Geometry: final body of the model. Coordinates: model frame, mm. Face numbers are marked on the shaded views. A direction names the side the tool comes from. Give positions to 0.01 mm unless a question says otherwise; leave off trailing zeros. Loops run counter-clockwise (first coordinate to the right, second up) from the corner with the lowest first, then second, coordinate; pieces in that order, holes last. Notation, with made-up numbers: (8.5, 41) - (53.5, 41) arc R11 cw to (53.5, 61) - close; hole circle Ø6 at (32, 41.5). An arc over 180 degrees is marked (long way). Use one line per item in the form item = value.
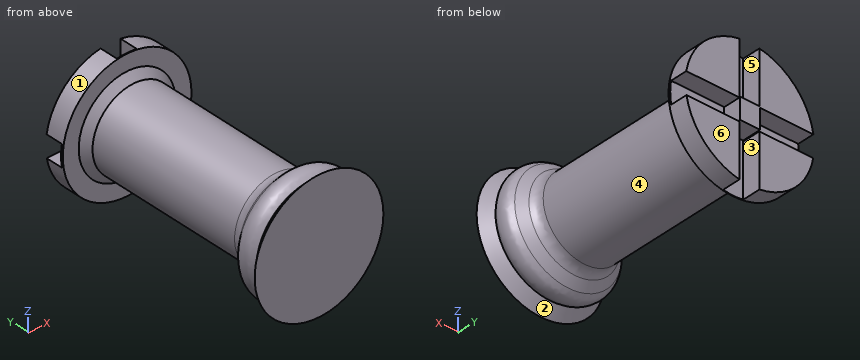
```python
from build123d import *

# Parameters (mm, degrees)
F2_R     = 5.08
F3_SIZE  = 2.54
F4_W     = 6.907339
F4_H     = 51.517231
F5_DEPTH = 6.35
F6_W     = 52.092841
F6_H     = 7.48295
F7_DEPTH = 5.9436
F8_W     = 6.907339
F8_H     = 7.284426
F9_DEPTH = 6.604


with BuildPart() as f1:
    # F0 (on Top) → F1 (revolve)
    with BuildSketch(Plane.XY):
        Polygon((22.304947, 47.919661), (0, 47.919661), (0, -33.52937), (22.304947, -33.52937), (18.717232, -30.197919), (22.304947, -26.334228), (14.246386, -18.851276), (14.246386, 41.300129), (22.304947, 41.300129), align=None)
    revolve(axis=Axis((0, 7.195146, 0), (0, -1, 0)))

    # F2
    f2_edges = [f1.edges().sort_by_distance(p)[0] for p in [
        (-22.304947, -26.334228, 0),
        (-14.246386, -18.851276, 0),
    ]]
    fillet(f2_edges, radius=F2_R)

    # F3
    f3_edges = [f1.edges().sort_by_distance(p)[0] for p in [
        (14.246386, 12.332043, 0),
        (-14.246383, -16.636044, 0),
        (-14.246386, 41.300129, 0),
    ]]
    chamfer(f3_edges, length=F3_SIZE)

    # F4 (on face) → F5 (cut)
    with BuildSketch(Plane(origin=(0, 47.919661, 0), x_dir=(-1, 0, 0), z_dir=(0, 1, 0))):
        with Locations((-0.143903, 0.575613)):
            Rectangle(F4_W, F4_H)
    extrude(amount=-F5_DEPTH, mode=Mode.SUBTRACT)

    # F6 (on face) → F7 (cut)
    with BuildSketch(Plane(origin=(0, 47.919661, 0), x_dir=(-1, 0, 0), z_dir=(0, 1, 0))):
        with Locations((0.287805, -0.143903)):
            Rectangle(F6_W, F6_H)
    extrude(amount=-F7_DEPTH, mode=Mode.SUBTRACT)

    # F8 (on face) → F9 (join)
    with BuildSketch(Plane(origin=(0, 41.569661, 0), x_dir=(-1, 0, 0), z_dir=(0, 1, 0))):
        with Locations((-0.143903, 0.12047)):
            Rectangle(F8_W, F8_H)
    extrude(amount=F9_DEPTH)


solid = f1.part
```
(1) Material intervals for L1, parallel to Y at x = -1, z = 6.5; L2, parallel to Y at x = -19, z = 2.5; L3, parallel to Y at x = -11.5, z = -3, sorted ascending. Write a range as from..to.
Solution:
L1 = -33.53..41.57
L2 = -33.53..-30.61, -29.68..-23.52, 41.3..41.98
L3 = -33.53..41.98
(2) Pin query (flat end, axial travel): P1, Ø1.5, axis at y = 18.5, z = -3, coming from the +X side; P2, Ø10, axis at x = 15, z = 1.5, coming from the +Y side; P3, Ø1, axis at x = 2.5, z = -5, coming from the +Y side. Return the tip coordinate at first contact, or that it passes through.
Solution:
P1 = 14.07
P2 = 47.92
P3 = 41.57
(3) Cut plane A-A (y = 2). Return the cut outline in (x, z), plus the area to 3 significant figures.
Solution:
outline = circle Ø28.49 at (0, 0)
area = 638 mm2
(4) Pull-direction query (X, two-part tool) for the marked faces 3, 4, 5 and 6; classes: released by +X, released by -X, zero draft, split by the parting line, or undercut.
Solution:
face_3 = undercut
face_4 = split by the parting line
face_5 = undercut
face_6 = zero draft
(5) Access query for the marked faces 1 and 2. Directions: +Z, -Z, +X, -X, +Y, -Y. A direction counts if a zero-diameter tool reaches every point of the face in a straight line with its end or side. Return the directions, or none.
Solution:
face_1 = +Y, -Y
face_2 = none
